```python
from build123d import *

# Parameters (mm, degrees)
SKETCH2_W           = 241.3
SKETCH2_H           = 228.6
SKETCH2_R           = 100
SKETCH2_R_2         = 72.5
BOSS_EXTRUDE1_DEPTH = 3.175


with BuildPart() as part:
    # Sketch2 → Boss-Extrude1 (new body)
    # profile 1 of 2: a face of its own
    with BuildSketch(Plane.XY):
        with Locations((-6.35, 0)):
            Rectangle(SKETCH2_W, SKETCH2_H)
        Circle(SKETCH2_R, mode=Mode.SUBTRACT)
    # profile 2 of 2: a face of its own
    with BuildSketch(Plane.XY):
        Circle(SKETCH2_R)
        Circle(SKETCH2_R_2, mode=Mode.SUBTRACT)
    extrude(amount=BOSS_EXTRUDE1_DEPTH)


solid = part.part
```
For this review, take the finished solid that the model builds, in its own axes (mm). Coordinates: 2 decimals unless noted, no trailing zeros. Write each loop counter-clockwise with the first axis right and the second up, starting at its lowest first coordinate (ties: lowest second). Pieces come first, ordered by that corner, then holes.
(1) The part is to be moulded in two halves that separate along Y. For faces 1 (the face through (-62, -49, 3.175)), 2 (the face through (69.15, 21.78, 1.57)), say which applies: +Y half, -Y half, draft (parallel to the pull), parting line (faces both ways), or undercut.
(2) Add section C-C on z = 0.9. Give the boundary of the cut face in (x, y), then the cut area to 3 significant figures.
(3) Add section B-B on x = 8.5. Give the boundary of the cut face in (y, z) (3 decimals).
(4) Add section A-A on y = 8.5. Give the boundary of the cut face in (x, z) (3 decimals), then the cut area to 3 significant figures.
(5) Wall thickness on probe 1 along Y at (x, z) = (0, 1.3); probe 2 along Y at (x, z) = (23.5, 2.95); probe 3 along X at (y, z) = (-10, 2.7): over which ranges is each line inside the solid? List them lowest first.
Answer sheet:
1. face 1: draft
1. face 2: undercut
2. outline: (-127, -114.3) - (114.3, -114.3) - (114.3, 114.3) - (-127, 114.3) - close; hole circle Ø145 at (0, 0)
2. area: 38,600 mm2
3. outline: (-114.3, 0) - (-72, 0) - (-72, 3.175) - (-114.3, 3.175) - close; (72, 0) - (114.3, 0) - (114.3, 3.175) - (72, 3.175) - close
4. outline: (-127, 0) - (-72, 0) - (-72, 3.175) - (-127, 3.175) - close; (72, 0) - (114.3, 0) - (114.3, 3.175) - (72, 3.175) - close
4. area: 309 mm2
5. probe 1: y = -114.3 to -72.5, 72.5 to 114.3
5. probe 2: y = -114.3 to -68.59, 68.59 to 114.3
5. probe 3: x = -127 to -71.81, 71.81 to 114.3
